Check sheet for the modelled part. Datum: model origin and axes. Units: mm. Coordinates: 2 decimals unless noted, no trailing zeros. Loops run counter-clockwise (first coordinate to the right, second up) from the corner with the lowest first, then second, coordinate; pieces in that order, holes last. Notation, with made-up numbers: M 86,24 L 126,24 A29 ccw 126,56 Z; hole C 46.5,75 d1. An arc over 180 degrees is marked long. Use CSV: the item, a comma, the result in double quotes. Start each with the question number.
(1) Scan lines: line 1 (Z direction, x = 0, y = 708.5); line 2 (Y direction, x = 5.5, z = -0.75). Record each from-to range of solid material in increasing order.
(2) Section check A-A on y = 443. Record the cut outline in (x, z), and give its area (3 significant figures).
(3) Go/stop test with flat-tipped pins: pin 1 Ø6.5 at (y, z) = (637.863, 0) entering from +X; pin 2 Ø9 at (y, z) = (637.863, 0) entering from +X. Record where each tip stops, or that it passes through.
Autodesk Inventor part; units mm, degrees
ref_plane "YZ Plane" through (0, 0, 0) normal (1, 0, 0) x (0, 1, 0)
ref_plane "XZ Plane" through (0, 0, 0) normal (0, 1, 0) x (-1, 0, 0)
ref_plane "XY Plane" through (0, 0, 0) normal (0, 0, 1) x (1, 0, 0)
sketch "Boceto1" plane through (0, 0, 0) normal (0, 1, 0) x (-1, 0, 0)
  line L0 (15, 15) -> (-15, 15)
  line L1 (-15, 15) -> (-15, -15)
  line L2 (-15, -15) -> (15, -15)
  line L3 (15, -15) -> (15, 15)
  line L4 (15, 15) -> (-15, -15) construction
  circle A0 centre (0, 0) radius 4
  dimension "d0" = 30
  dimension "d1" = 8
extrude "Extrusión1" add sketch "Boceto1" along normal blind 736
sketch "Sketch2" plane through (15, 0, 15) normal (1, 0, 0) x (0, 0, -1)
  line L0 (0, 736) -> (30, 736)
  circle A0 centre (15, 637.863) radius 4
  point P0 (15, 0)
  dimension "d5" = 8
extrude "Extrusion2" cut sketch "Sketch2" against normal blind 30
properties part number "P_3030_1500"
Outcome:
1,line 1,"z = -15 to -4, 4 to 15"
1,line 2,"y = 0 to 633.93, 641.79 to 736"
2,outline,"M -15,-15 L 15,-15 L 15,15 L -15,15 Z; hole C 0,0 d8"
2,area,"850 mm²"
3,pin 1,"passes through"
3,pin 2,"stops at x = 15"
